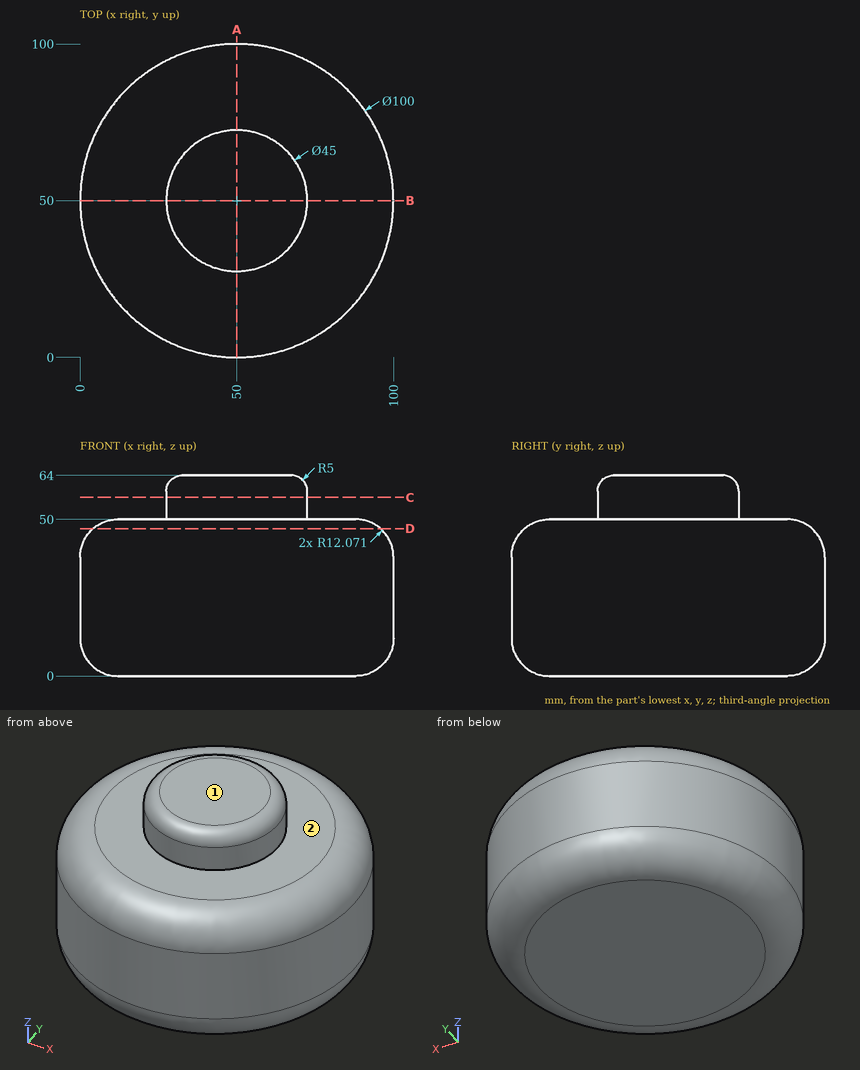
For this review, use the dimensioned drawing (mm, ordinates from the lowest corner) and the shaded views. A direction names the side the tool comes from. Coordinates: 2 decimals unless noted, no trailing zeros. Write each loop counter-clockwise with the first axis right and the second up, starting at its lowest first coordinate (ties: lowest second). Pieces come first, ordered by that corner, then holes. Notation, with made-up numbers: (44.25, 29) - (85.25, 29) arc R34 ccw to (85.25, 59) - close; hole circle Ø4 at (0, 66.5). An arc over 180 degrees is marked (long way). Answer in a Markdown table with one row per item. Add a question column.
Q1. For the marked faces 1 and 2, list the 3-axis set-ups (+Z, -Z, +X, -X, +Y, -Y) from which the entire face can be reached by the end or side of a thin tool; tool diameter is ignored.
Q2. Clearance check with flat-ended pins moving along their axes: pin 1 (3 mm diameter, centred on x = 89, z = 7.5, fed in from -Y); pin 2 (6 mm diameter, centred on x = 59.5, z = 48, fed in from +Y); pin 3 (1 mm diameter, centred on x = 47, y = 26, fed in from +Z). State where each tip first meets the part, or that it passes through.
Q3. To check wall thickness, follow line 1 along Z through (x, y) = (49.5, 85); line 2 along X through (y, z) = (50.5, 16.5); line 3 along Z through (x, y) = (39.5, 95). State the ranges of each line that lie inside material, in increasing order. Write a range as from..to.
Q4. Consider section A-A on x = 50. Give the boundary of the cut face in (y, z).
Q5. Consider section C-C on z = 57. Give the boundary of the cut face in (x, y), then the cut area to 3 significant figures.
Q6. Consider section D-D on z = 47. Give the boundary of the cut face in (x, y), then the cut area to 3 significant figures.
Answers below:
| question | item | result |
|---|---|---|
| 1 | face 1 | +Z, +X, -X, +Y, -Y |
| 1 | face 2 | +Z |
| 2 | pin 1 | y = 18.1 |
| 2 | pin 2 | y = 96.83 |
| 2 | pin 3 | z = 50 |
| 3 | line 1 | 0..50 |
| 3 | line 2 | 0..100 |
| 3 | line 3 | 3.29..46.71 |
| 4 | outline | (0, 12.07) arc R12.07 ccw to (12.07, 0) - (87.93, 0) arc R12.07 ccw to (100, 12.07) - (100, 37.93) arc R12.07 ccw to (87.93, 50) - (72.5, 50) - (72.5, 59) arc R5 ccw to (67.5, 64) - (32.5, 64) arc R5 ccw to (27.5, 59) - (27.5, 50) - (12.07, 50) arc R12.07 ccw to (0, 37.93) - close |
| 5 | outline | circle Ø45 at (50, 50) |
| 5 | area | 1,590 mm² |
| 6 | outline | circle Ø91.79 at (50, 50) |
| 6 | area | 6,620 mm² |
